Part model, mm, in its own coordinate system. Coordinates: 2 decimals unless noted, no trailing zeros. Loops run counter-clockwise (first coordinate to the right, second up) from the corner with the lowest first, then second, coordinate; pieces in that order, holes last. Notation, with made-up numbers: (65.5, 75) - (108.5, 75) arc R20 cw to (108.5, 111) - close; hole circle Ø8 at (21.5, 51). An arc over 180 degrees is marked (long way). Use a Markdown table: item, result. Add a question column.
1. Wall check: probe 1 along X at (y, z) = (1.15, 0); probe 2 along X at (y, z) = (0.6, 0.25); probe 3 along Z at (x, y) = (5, 1). Give the ranges that are in metal, low to high. Write a range as [from, to].
2. Band-saw the part on B-B, the plane z = 0. Give the cut face in (x, y), plus the area to 3 significant figures.
3. Band-saw the part on A-A, the plane y = 1.8. Give the cut face in (x, z).
4. Drop a flat-ended pin along its axis: pin 1 (3 mm diameter, centred on y = 3, z = -4.5, fed in from +X). Give the stop position or say it passes through.
5. Pull direction X, two halves, no side cores. Call faces 1 (the flat face through (5.846, 2.465, -3.719)), 2 (the flat face through (-1.2, 5, -6.4)), 3 (the flat face through (-6.144, 2.465, -3.203)), 4 (the cylindrical face through (-1.38, 2.46, 6.2)): pulls with the +X half, pulls with the -X half, needs draft (parallel to the pull), parting line crosses it, or undercut.
from build123d import *

# Parameters (mm, degrees)
SKETCH4_R           = 6.35
BOSS_EXTRUDE1_DEPTH = 5
SKETCH9_OUTSIDE_W   = 43.162
SKETCH9_OUTSIDE_H   = 41.428
SKETCH9_OUTSIDE_R   = 6.92820323
CUT_EXTRUDE1_DEPTH  = 6
CUT_EXTRUDE1_TAPER  = 60


with BuildPart() as part:
    # Sketch4 → Boss-Extrude1 (new body)
    with BuildSketch(Plane(origin=(0, 0, 0), x_dir=(1, 0, 0), z_dir=(0, 1, 0))):
        Polygon((3.640964438, 7.123438633), (-4.348596599, 6.714887014), (-7.989561038, -0.408551619), (-3.640964438, -7.123438633), (4.348596599, -6.714887014), (7.989561038, 0.408551619), align=None)
        Circle(SKETCH4_R, mode=Mode.SUBTRACT)
    extrude(amount=BOSS_EXTRUDE1_DEPTH)

    # Sketch9 outside → Cut-Extrude1 (cut, through all)
    with BuildSketch(Plane.XZ):
        Rectangle(SKETCH9_OUTSIDE_W, SKETCH9_OUTSIDE_H)
        Circle(SKETCH9_OUTSIDE_R, mode=Mode.SUBTRACT)
    extrude(amount=-CUT_EXTRUDE1_DEPTH, taper=CUT_EXTRUDE1_TAPER, mode=Mode.SUBTRACT)


solid = part.part
Geometry check:
| question | item | result |
|---|---|---|
| 1 | probe 1 | x = [-7.78, -6.35], [6.35, 7.78] |
| 1 | probe 2 | x = [-7.91, -6.35], [6.35, 7.65] |
| 1 | probe 3 | z = [-5.02, -3.91], [3.91, 5.44] |
| 2 | outline | (-7.78, 0.49) - (-6.93, 0) - (-6.35, 0) - (-6.35, 5) - (-7.78, 5) - close; (6.35, 0) - (6.93, 0) - (7.78, 0.49) - (7.78, 5) - (6.35, 5) - close |
| 2 | area | 13.9 mm^2 |
| 3 | outline | (-7.99, 0.41) - (-4.35, -6.71) - (3.64, -7.12) - (7.99, -0.41) - (4.35, 6.71) - (-3.64, 7.12) - close; hole circle Ø12.7 at (0, 0) |
| 4 | pin 1 | stops at x = 6.31 |
| 5 | face 1 | pulls with the +X half |
| 5 | face 2 | needs draft |
| 5 | face 3 | pulls with the -X half |
| 5 | face 4 | undercut |
